```python
from build123d import *

# Parameters (mm, degrees)
PAD001_DEPTH = 10
PAD002_DEPTH = 10
SKETCH004_R  = 5
PAD003_DEPTH = 10
PAD_DEPTH    = 96
POCKET_DEPTH = 60.001


with BuildPart() as pad001:
    # Sketch002 → Pad001 (new body)
    with BuildSketch(Plane.YZ):
        Polygon((30, 30), (-26.547005, 30), (-15, 50), (30, 50), align=None)
    extrude(amount=PAD001_DEPTH)


with BuildPart() as pad003:
    # Sketch003 → Pad002 (new body)
    with BuildSketch(Plane.XZ.offset(-30)):
        Polygon((10, 50), (10, 30), (64, 30), (44, 50), align=None)
    extrude(amount=PAD002_DEPTH)

    # Sketch004 → Pad003 (new body)
    with BuildSketch(Plane(origin=(0, 30, 50), x_dir=(-1, 0, 0), z_dir=(0, 0, 1))):
        Polygon((0, 0), (0, 45), (-24, 45), (-44, 21.164928), (-44, 0), align=None)
        with Locations((-24, 24)):
            Circle(SKETCH004_R, mode=Mode.SUBTRACT)
    extrude(amount=PAD003_DEPTH)


with BuildPart() as fusion:
    # Sketch → Pad (new body)
    with BuildSketch(Plane.YZ):
        Polygon((-18, 0), (18, 0), (18, 10), (12, 10), (12, 18), (30, 18), (30, 30), (-30, 30), (-30, 18), (-12, 18), (-12, 10), (-18, 10), align=None)
    extrude(amount=PAD_DEPTH)

    # Sketch001 → Pocket (cut, through all)
    with BuildSketch(Plane(origin=(0, -30, 0), x_dir=(0, 0, -1), z_dir=(0, -1, 0))):
        Polygon((-33.660889, 86), (-25, 86), (-25, 74), (-33.660889, 79.000366), align=None)
    extrude(amount=-POCKET_DEPTH, mode=Mode.SUBTRACT)

    # Fusion: union Pad001, Pad003
    add(pad001.part)
    add(pad003.part)


solid = fusion.part
```
CAD build for the part. Positions are in the model's coordinates, mm. A direction names the side the tool comes from. Round coordinates to 2 decimals unless told otherwise and drop trailing zeros. Loops run counter-clockwise (first coordinate to the right, second up) from the corner with the lowest first, then second, coordinate; pieces in that order, holes last. Notation, with made-up numbers: M -23.5,78.5 L 1.5,78.5 A13 ccw 1.5,82.5 Z; hole C 2,-7.75 d3. An arc over 180 degrees is marked long. Use a Markdown table: item, result. Add a question column.
(1) Cut at D-D (y = -1). Give the cut face in (x, z).
(2) Cut at A-A (z = 52.5). Give the cut face in (x, y), and give its area (3 significant figures).
(3) Pull direction X, two halves, no side cores. Call faces 4 (the face through (29, 6, 55)), 5 (the face through (47, -18, 5)), 6 (the face through (44, 19, 55)): +X half, -X half, draft (parallel to the pull), parting line (faces both ways), or undercut.
(4) Drill centre lines: line 1 (Z direction, x = 83.5, y = 16.5); line 2 (Z direction, x = 34.5, y = 19); line 3 (Y direction, x = 24, z = 53.5). Where is each one in solid material? Low to high.
(5) Which spindle directions (+Z, -Z, +X, -X, +Y, -Y) get a long thin tool onto all of the face, cutting with end or side? Do faces 1 (the face through (47, -15, 10)), 2 (the face through (20, 2, 50)), 3 (the face through (91, 0, 30)). Say none if no direction does.
(6) Cut at C-C (y = -16.5). Give the cut face in (x, z), and give its area (3 significant figures).
(7) Flat gauge pins, fed straight in: pin 1 (1.8 mm diameter, centred on x = 44.5, y = -16.5, fed in from +Z); pin 2 (10 mm diameter, centred on x = 50, z = 42.5, fed in from -Y); pin 3 (6.5 mm diameter, centred on x = 63, z = 14, fed in from +Y). Where does each tip first touch, or does it go through?
(8) Cut at B-B (x = 52). Give the cut face in (y, z), and give its area (3 significant figures).
Geometry says:
| question | item | result |
|---|---|---|
| 1 | outline | M 0,0 L 96,0 L 96,30 L 86,30 L 86,25 L 74,25 L 76.89,30 L 10,30 L 10,50 L 35.75,50 L 35.75,60 L 0,60 Z |
| 2 | outline | M 0,-15 L 24,-15 L 44,8.84 L 44,30 L 0,30 Z; hole C 24,6 d10 |
| 2 | area | 1,660 mm² |
| 3 | face 4 | undercut |
| 3 | face 5 | draft |
| 3 | face 6 | +X half |
| 4 | line 1 | z = 0 to 10, 18 to 25 |
| 4 | line 2 | z = 18 to 30, 50 to 60 |
| 4 | line 3 | y = -15 to 1, 11 to 30 |
| 5 | face 1 | +X, -X, -Y |
| 5 | face 2 | +X, -Y |
| 5 | face 3 | +Z, +X, +Y, -Y |
| 6 | outline | M 0,0 L 96,0 L 96,10 L 0,10 Z; M 0,18 L 96,18 L 96,30 L 86,30 L 86,25 L 74,25 L 76.89,30 L 10,30 L 10,47.4 L 0,47.4 Z |
| 6 | area | 2,230 mm² |
| 7 | pin 1 | stops at z = 30 |
| 7 | pin 2 | stops at y = 20 |
| 7 | pin 3 | stops at y = 12 |
| 8 | outline | M -30,18 L -12,18 L -12,10 L -18,10 L -18,0 L 18,0 L 18,10 L 12,10 L 12,18 L 30,18 L 30,42 L 20,42 L 20,30 L -30,30 Z |
| 8 | area | 1,390 mm² |
